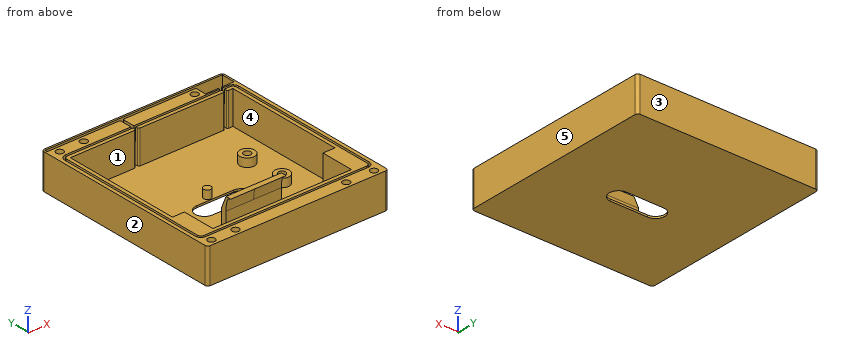
```python
from build123d import *

# Parameters (mm, degrees)
PAD_DEPTH       = 1
PAD001_DEPTH    = 19
SKETCH002_R     = 4
SKETCH002_R_2   = 1.95
SKETCH002_R_3   = 2
PAD002_DEPTH    = 5.5
PAD003_DEPTH    = 15
POCKET_DEPTH    = 7
PAD004_DEPTH    = 1
SKETCH007_R     = 1.95
POCKET001_DEPTH = 5
PAD014_DEPTH    = 1


with BuildPart() as part:
    # Sketch → Pad (new body)
    with BuildSketch(Plane.XY):
        with BuildLine():
            Line((-47.5, -52.5), (47.5, -52.5))
            ThreePointArc((47.5, -52.5), (48.56066, -52.06066), (49, -51))
            Line((49, -51), (49, 51))
            ThreePointArc((49, 51), (48.56066, 52.06066), (47.5, 52.5))
            Line((47.5, 52.5), (-47.5, 52.5))
            ThreePointArc((-47.5, 52.5), (-48.56066, 52.06066), (-49, 51))
            Line((-49, 51), (-49, -51))
            ThreePointArc((-49, -51), (-48.56066, -52.06066), (-47.5, -52.5))
        make_face()
        with BuildLine():
            ThreePointArc((-10, 0), (-15, -5), (-10, -10))
            Line((-10, -10), (10, -10))
            ThreePointArc((10, -10), (15, -5), (10, 0))
            Line((-10, 0), (10, 0))
        make_face(mode=Mode.SUBTRACT)
    extrude(amount=PAD_DEPTH)

    # Sketch001 → Pad001 (join)
    with BuildSketch(Plane.XY):
        with BuildLine():
            Line((-47.5, -52.5), (47.5, -52.5))
            ThreePointArc((47.5, -52.5), (48.56066, -52.06066), (49, -51))
            Line((49, -51), (49, 51))
            ThreePointArc((49, 51), (48.56066, 52.06066), (47.5, 52.5))
            Line((47.5, 52.5), (-47.5, 52.5))
            ThreePointArc((-47.5, 52.5), (-48.56066, 52.06066), (-49, 51))
            Line((-49, 51), (-49, -51))
            ThreePointArc((-49, -51), (-48.56066, -52.06066), (-47.5, -52.5))
        make_face()
        with BuildLine():
            Line((44, 40.1), (44, -24.5))
            Line((44, -24.5), (37.5, -24.5))
            Line((37.5, -24.5), (37.5, -42.5))
            Line((37.5, -42.5), (-37.5, -42.5))
            Line((-37.5, -42.5), (-37.5, -24.5))
            Line((-37.5, -24.5), (-44, -24.5))
            Line((-44, -24.5), (-44, 40.1))
            Line((-44, 40.1), (-9.25, 40.1))
            ThreePointArc((-9.25, 40.1), (-8.71967, 40.31967), (-8.5, 40.85))
            Line((-8.5, 40.85), (-8.5, 49.35))
            ThreePointArc((-8.5, 49.35), (-8.71967, 49.88033), (-9.25, 50.1))
            Line((-9.25, 50.1), (-48, 50.1))
            Line((-48, 50.1), (-48, 51.5))
            Line((-48, 51.5), (48, 51.5))
            Line((48, 44), (48, 51.5))
            Line((48, 44), (41.5, 44))
            ThreePointArc((41.5, 44), (41.146447, 43.853553), (41, 43.5))
            Line((41, 43.5), (41, 40.6))
            ThreePointArc((41, 40.6), (41.146447, 40.246447), (41.5, 40.1))
            Line((41.5, 40.1), (44, 40.1))
        make_face(mode=Mode.SUBTRACT)
        with BuildLine():
            Line((-7, 40.85), (-7, 49.35))
            ThreePointArc((-6.25, 50.1), (-6.78033, 49.88033), (-7, 49.35))
            Line((-6.25, 50.1), (32.5, 50.1))
            Line((32.5, 50.1), (32.5, 44))
            Line((32.5, 44), (39, 44))
            ThreePointArc((39.5, 43.5), (39.353553, 43.853553), (39, 44))
            Line((39.5, 43.5), (39.5, 40.6))
            ThreePointArc((39, 40.1), (39.353553, 40.246447), (39.5, 40.6))
            Line((39, 40.1), (-6.25, 40.1))
            ThreePointArc((-7, 40.85), (-6.78033, 40.31967), (-6.25, 40.1))
        make_face()
    extrude(amount=PAD001_DEPTH)

    # Sketch002 → Pad002 (join)
    with BuildSketch(Plane.XY):
        with Locations((29, 13.5)):
            Circle(SKETCH002_R)
        with Locations((29, 13.5)):
            Circle(SKETCH002_R_2, mode=Mode.SUBTRACT)
        with Locations((29, -8.5)):
            Circle(SKETCH002_R)
        with Locations((29, -8.5)):
            Circle(SKETCH002_R_2, mode=Mode.SUBTRACT)
        with Locations((-2, 2.5)):
            Circle(SKETCH002_R_3)
    extrude(amount=PAD002_DEPTH)

    # Sketch003 → Pad003 (join, symmetric)
    with BuildSketch(Plane.YZ):
        with BuildLine():
            Line((-24.5, 0), (-24.5, 11))
            add(Edge.make_bspline(
                [(-27.5, 18), (-24.5, 18), (-24.5, 11)],
                knots=[0, 0, 0, 1, 1, 1], degree=2))
            Line((-27.5, 18), (-24.5, 18))
            Line((-24.5, 18), (-21.5, 11))
            Line((-21.5, 11), (-21.5, 0))
            Line((-21.5, 0), (-24.5, 0))
        make_face()
    extrude(amount=PAD003_DEPTH, both=True)

    # Sketch004 (on Face14 of Pad003) → Pocket (cut)
    with BuildSketch(Plane.XY.offset(19)):
        with BuildLine():
            Line((47.1, -42.5), (47.1, 40.1))
            ThreePointArc((47.1, 40.1), (46.192031, 42.292031), (44, 43.2))
            Line((44, 43.2), (-44, 43.2))
            ThreePointArc((-44, 43.2), (-46.192031, 42.292031), (-47.1, 40.1))
            Line((-47.1, 40.1), (-47.1, -42.5))
            ThreePointArc((-47.1, -42.5), (-46.192031, -44.692031), (-44, -45.6))
            Line((-44, -45.6), (44, -45.6))
            ThreePointArc((44, -45.6), (46.192031, -44.692031), (47.1, -42.5))
        make_face()
        with BuildLine():
            Line((45.9, -42.5), (45.9, 40.1))
            ThreePointArc((45.9, 40.1), (45.343503, 41.443503), (44, 42))
            Line((44, 42), (-44, 42))
            ThreePointArc((-44, 42), (-45.343503, 41.443503), (-45.9, 40.1))
            Line((-45.9, 40.1), (-45.9, -42.5))
            ThreePointArc((-45.9, -42.5), (-45.343503, -43.843503), (-44, -44.4))
            Line((-44, -44.4), (44, -44.4))
            ThreePointArc((44, -44.4), (45.343503, -43.843503), (45.9, -42.5))
        make_face(mode=Mode.SUBTRACT)
    extrude(amount=-POCKET_DEPTH, mode=Mode.SUBTRACT)

    # Sketch005 → Pad004 (join)
    with BuildSketch(Plane.YZ.offset(36.5)):
        Polygon((-24.5, 0), (-24.5, 4), (-38.5, 4), (-38.5, 15), (-42.5, 15), (-42.5, 0), align=None)
    extrude(amount=PAD004_DEPTH)

    # Sketch007 (on DatumPlane) → Pocket001 (cut)
    with BuildSketch(Plane.XY.offset(19)):
        with Locations((-44, -49.166667)):
            Circle(SKETCH007_R)
        with Locations((44, -49.166667)):
            Circle(SKETCH007_R)
        with Locations((-44, 46.766667)):
            Circle(SKETCH007_R)
        with Locations((29, 46.766667)):
            Circle(SKETCH007_R)
        with Locations((-31, 46.766667)):
            Circle(SKETCH007_R)
        with Locations((29, -49.166667)):
            Circle(SKETCH007_R)
        with Locations((-31, -49.166667)):
            Circle(SKETCH007_R)
    extrude(amount=-POCKET001_DEPTH, mode=Mode.SUBTRACT)

    # Sketch006 → Pad014 (join)
    with BuildSketch(Plane.YZ.offset(-37.5)):
        Polygon((-42.5, 0), (-42.5, 15), (-38.5, 15), (-38.5, 4), (-24.5, 4), (-24.5, 0), align=None)
    extrude(amount=PAD014_DEPTH)


solid = part.part
```
Build history of the part. All positions in model axes, mm. Face numbers are marked on the shaded views. A direction names the side the tool comes from. Round coordinates to 2 decimals unless told otherwise and drop trailing zeros. Loops run counter-clockwise (first coordinate to the right, second up) from the corner with the lowest first, then second, coordinate; pieces in that order, holes last.
Item 1: Saw through at A-A (z = 7.5). State how many separate pieces and enclosed holes the cut face has, then the cut area to 3 significant figures.
Item 2: Pin check, flat tips, straight feed: P1, Ø1.2, axis at x = -43.5, y = 47.5, coming from the +Z side; P2, Ø6, axis at x = -24.5, y = 21, coming from the +Z side; P3, Ø4.5, axis at x = 29.5, y = -8.5, coming from the +Z side. Stop position of each tip, or through.
Item 3: Saw through at D-D (y = -8.5). List the corners of the cut face in (x, z), then the cut area to 3 significant figures.
Item 4: Saw through at B-B (x = -18). List the corners of the cut face in (y, z).
Item 5: Drill centre lines: line 1 along X through (y, z) = (13.5, 2); line 2 along Y through (x, z) = (24.5, 15.5); line 3 along Y through (x, z) = (-0.5, 7.5). Where is each one in solid material? Low to high.
Item 6: Which spindle directions (+Z, -Z, +X, -X, +Y, -Y) get a long thin tool onto all of the face, cutting with end or side? Do the marked faces 4 and 5. Say none if no direction does.
Item 7: Two-plate mould, pull along X, no slides. Class the marked faces 1, 2 and 3: released by +X, released by -X, zero draft, split by the parting line, or undercut.
Item 8: Saw through at C-C (y = 28.5). List the corners of the cut face in (x, z), then the cut area to 3 significant figures.
Worked answers:
1. separate pieces: 3
1. enclosed holes: 1
1. area: 3,100 mm2
2. P1: stops at z = 14
2. P2: stops at z = 1
2. P3: stops at z = 5.5
3. outline: (-49, 0) - (-13.57, 0) - (-13.57, 1) - (-44, 1) - (-44, 19) - (-45.9, 19) - (-45.9, 12) - (-47.1, 12) - (-47.1, 19) - (-49, 19) - close; (13.57, 0) - (49, 0) - (49, 19) - (47.1, 19) - (47.1, 12) - (45.9, 12) - (45.9, 19) - (44, 19) - (44, 1) - (33, 1) - (33, 5.5) - (30.95, 5.5) - (30.95, 1) - (27.05, 1) - (27.05, 5.5) - (25, 5.5) - (25, 1) - (13.57, 1) - close
3. area: 253 mm2
4. outline: (-52.5, 0) - (52.5, 0) - (52.5, 19) - (51.5, 19) - (51.5, 1) - (50.1, 1) - (50.1, 19) - (43.2, 19) - (43.2, 12) - (42, 12) - (42, 19) - (40.1, 19) - (40.1, 1) - (-42.5, 1) - (-42.5, 19) - (-44.4, 19) - (-44.4, 12) - (-45.6, 12) - (-45.6, 19) - (-52.5, 19) - close
5. line 1: x = -49 to -44, 25 to 27.05, 30.95 to 33, 44 to 49
5. line 2: y = -52.5 to -45.6, -44.4 to -42.5, 40.1 to 42, 43.2 to 50.1, 51.5 to 52.5
5. line 3: y = -52.5 to -42.5, -24.5 to -21.5, 40.1 to 50.1, 51.5 to 52.5
6. face 4: +Z
6. face 5: +Z, -Z, +X, +Y, -Y
7. face 1: undercut
7. face 2: released by -X
7. face 3: zero draft
8. outline: (-49, 0) - (49, 0) - (49, 19) - (47.1, 19) - (47.1, 12) - (45.9, 12) - (45.9, 19) - (44, 19) - (44, 1) - (-44, 1) - (-44, 19) - (-45.9, 19) - (-45.9, 12) - (-47.1, 12) - (-47.1, 19) - (-49, 19) - close
8. area: 261 mm2
